Geometry: final body of the model. Coordinates: model frame, mm. A direction names the side the tool comes from. Give positions to 0.01 mm unless a question says otherwise; leave off trailing zeros. Loops run counter-clockwise (first coordinate to the right, second up) from the corner with the lowest first, then second, coordinate; pieces in that order, holes last.
from build123d import *

# Parameters (mm, degrees)
EXTRUDE_1_DEPTH = 10


with BuildPart() as part:
    # 草图1 → 凸台-拉伸1 (new body)
    with BuildSketch(Plane(origin=(0, 0, 0), x_dir=(1, 0, 0), z_dir=(0, 1, 0))):
        with BuildLine():
            Line((59.993482859, 52.922415047), (17.67766953, 10.606601718))
            ThreePointArc((17.67766953, 10.606601718), (10.606601718, 10.606601718), (10.606601718, 17.67766953))
            Line((10.606601718, 17.67766953), (52.922415047, 59.993482859))
            ThreePointArc((52.922415047, 59.993482859), (51.012147139, 61.625975402), (49.05155132, 63.197668573))
            ThreePointArc((49.05155132, 63.197668573), (0, 43.137085), (-49.05155132, 63.197668573))
            ThreePointArc((-49.05155132, 63.197668573), (-51.012147139, 61.625975402), (-52.922415047, 59.993482859))
            Line((-52.922415047, 59.993482859), (-10.606601718, 17.67766953))
            ThreePointArc((-10.606601718, 17.67766953), (-10.606601718, 10.606601718), (-17.67766953, 10.606601718))
            Line((-17.67766953, 10.606601718), (-59.993482859, 52.922415047))
            ThreePointArc((-59.993482859, 52.922415047), (-61.625975402, 51.012147139), (-63.197668573, 49.05155132))
            ThreePointArc((-63.197668573, 49.05155132), (-43.137085, 0), (-63.197668573, -49.05155132))
            ThreePointArc((-63.197668573, -49.05155132), (-61.625975402, -51.012147139), (-59.993482859, -52.922415047))
            Line((-59.993482859, -52.922415047), (-17.67766953, -10.606601718))
            ThreePointArc((-17.67766953, -10.606601718), (-10.606601718, -10.606601718), (-10.606601718, -17.67766953))
            Line((-10.606601718, -17.67766953), (-52.922415047, -59.993482859))
            ThreePointArc((-52.922415047, -59.993482859), (-51.012147139, -61.625975402), (-49.05155132, -63.197668573))
            ThreePointArc((-49.05155132, -63.197668573), (0, -43.137085), (49.05155132, -63.197668573))
            ThreePointArc((49.05155132, -63.197668573), (51.012147139, -61.625975402), (52.922415047, -59.993482859))
            Line((52.922415047, -59.993482859), (10.606601718, -17.67766953))
            ThreePointArc((10.606601718, -17.67766953), (10.606601718, -10.606601718), (17.67766953, -10.606601718))
            Line((17.67766953, -10.606601718), (59.993482859, -52.922415047))
            ThreePointArc((59.993482859, -52.922415047), (61.625975402, -51.012147139), (63.197668573, -49.05155132))
            ThreePointArc((63.197668573, -49.05155132), (43.137085, 0), (63.197668573, 49.05155132))
            ThreePointArc((63.197668573, 49.05155132), (61.625975402, 51.012147139), (59.993482859, 52.922415047))
        make_face()
        with BuildLine():
            Line((-2, 9.797958971), (-2, 13.797958971))
            Line((-2, 13.797958971), (2, 13.797958971))
            Line((2, 13.797958971), (2, 9.797958971))
            ThreePointArc((2, 9.797958971), (0, -10), (-2, 9.797958971))
        make_face(mode=Mode.SUBTRACT)
    extrude(amount=EXTRUDE_1_DEPTH)


solid = part.part
Item 1: Section query D-D on z = -20.5. Return loops of the section in (x, y).
Values follow:
outline: (-46.21, 0) - (-27.57, 0) - (-27.57, 10) - (-46.21, 10) - close; (-13.43, 0) - (13.43, 0) - (13.43, 10) - (-13.43, 10) - close; (27.57, 0) - (46.21, 0) - (46.21, 10) - (27.57, 10) - close
Item 2: Pin query (flat end, axial travel): pin 1 (4.5 mm diameter, centred on y = 5, z = -11, fed in from -X); pin 2 (1.2 mm diameter, centred on y = 7, z = -12, fed in from +X); pin 3 (5 mm diameter, centred on x = -15.5, y = 8.5, fed in from -Z). Return the tip coordinate at first contact, or that it passes through.
Values follow:
pin 1: stops at x = -44.4
pin 2: stops at x = 44.28
pin 3: stops at z = -45.49
Item 3: Ray query, probe 1 along X at (y, z) = (8, 20); probe 2 along Z at (x, y) = (11.5, 1); probe 3 along X at (y, z) = (6.75, 17.5). Return the intervals inside material, ascending.
Values follow:
probe 1: x = -46.06 to -27.07, -12.93 to 12.93, 27.07 to 46.06
probe 2: z = -44.09 to -18.57, -9.9 to 9.9, 18.57 to 44.09
probe 3: x = -45.36 to -24.57, -10.44 to 10.44, 24.57 to 45.36
Item 4: Section query B-B on y = 8.5. Return loops of the section in (x, z).
Values follow:
outline: (-63.2, -49.05) arc R80 ccw to (-59.99, -52.92) - (-17.68, -10.61) arc R5 cw to (-10.61, -17.68) - (-52.92, -59.99) arc R80 ccw to (-49.05, -63.2) arc R70 cw to (49.05, -63.2) arc R80 ccw to (52.92, -59.99) - (10.61, -17.68) arc R5 cw to (17.68, -10.61) - (59.99, -52.92) arc R80 ccw to (63.2, -49.05) arc R70 cw to (63.2, 49.05) arc R80 ccw to (59.99, 52.92) - (17.68, 10.61) arc R5 cw to (10.61, 17.68) - (52.92, 59.99) arc R80 ccw to (49.05, 63.2) arc R70 cw to (-49.05, 63.2) arc R80 ccw to (-52.92, 59.99) - (-10.61, 17.68) arc R5 cw to (-17.68, 10.61) - (-59.99, 52.92) arc R80 ccw to (-63.2, 49.05) arc R70 cw to start; hole (-2, -13.8) - (2, -13.8) - (2, -9.8) arc R10 ccw (long way) to (-2, -9.8) - close
Item 5: Draft query along X for faces 1 (the face through (-32.06, 4.93, -39.13)), 2 (the face through (-61.648, 4.93, 50.985)), 3 (the face through (43.14, 4.93, 0.76)). Return one class per face: +X half, -X half, draft (parallel to the pull), parting line (faces both ways), or undercut.
Values follow:
face 1: undercut
face 2: -X half
face 3: +X half
Item 6: Section query A-A on z = 0. Return loops of the section in (x, y), plus the area to 3 significant figures.
Values follow:
outline: (-43.14, 0) - (-10, 0) - (-10, 10) - (-43.14, 10) - close; (10, 0) - (43.14, 0) - (43.14, 10) - (10, 10) - close
area: 663 mm2
Item 7: Section query C-C on x = 0. Return loops of the section in (y, z).
Values follow:
outline: (0, -43.14) - (10, -43.14) - (10, -13.8) - (0, -13.8) - close; (0, 10) - (10, 10) - (10, 43.14) - (0, 43.14) - close
Item 8: Set-up query: faces 4 (the face through (61.604, 4.93, 51.039)), 5 (the face through (-31.47, 4.93, 38.54)). Return all of +Z, -Z, +X, -X, +Y, -Y with unobstructed straight access to the full face (end or side cutting, diameter ignored); none if empty.
Values follow:
face 4: +Z, +X, +Y, -Y
face 5: +Y, -Y
